from build123d import *

# Parameters (mm, degrees)
SKETCH_1_W          = 40
SKETCH_1_H          = 16.8
EXTRUDE_1_DEPTH     = 1
SKETCH_3_R          = 1.6
SKETCH_3_R_2        = 2.55
SKETCH_3_W          = 12.882492612
SKETCH_3_H          = 6.05
CUT_EXTRUDE_1_DEPTH = 2


with BuildPart() as part:
    # Эскиз1 → Бобышка-Вытянуть1 (new body)
    with BuildSketch(Plane(origin=(0, 0, 0), x_dir=(1, 0, 0), z_dir=(0, 1, 0))):
        Rectangle(SKETCH_1_W, SKETCH_1_H)
    extrude(amount=EXTRUDE_1_DEPTH)

    # Эскиз3 → Вырез-Вытянуть1 (cut, through all)
    with BuildSketch(Plane(origin=(0, 1, 0), x_dir=(1, 0, 0), z_dir=(0, 1, 0))):
        with Locations((-15, -3)):
            Circle(SKETCH_3_R)
        with Locations((15, -3)):
            Circle(SKETCH_3_R)
        with Locations((0, 2.35)):
            Circle(SKETCH_3_R_2)
        with Locations((13.558753694, 5.375)):
            Rectangle(SKETCH_3_W, SKETCH_3_H)
        with Locations((-13.558753694, 5.375)):
            Rectangle(SKETCH_3_W, SKETCH_3_H)
    extrude(amount=-CUT_EXTRUDE_1_DEPTH, mode=Mode.SUBTRACT)


solid = part.part
Read the model definition and answer for the solid it produces. Units are mm, in the model's axes. A direction names the side the tool comes from. Give positions to 0.01 mm unless a question says otherwise; leave off trailing zeros. Loops run counter-clockwise (first coordinate to the right, second up) from the corner with the lowest first, then second, coordinate; pieces in that order, holes last. Notation, with made-up numbers: (34.5, 58) -> (64.5, 58) arc R20 ccw to (64.5, 91) -> close; hole circle Ø1 at (-29.75, 27.5). An arc over 180 degrees is marked (long way). Use a Markdown table: item, result.
Q1. Section D-D, the plane z = -2.75 is taken. Determine the outline of the cut face in (x, y).
Solved:
| item | result |
|---|---|
| outline | (-7.12, 0) -> (-2.52, 0) -> (-2.52, 1) -> (-7.12, 1) -> close; (2.52, 0) -> (7.12, 0) -> (7.12, 1) -> (2.52, 1) -> close |
Q2. A tool of negligible diameter and unlimited length cuts with its end or side. For faces 1 (the face through (7.118, 0.5, -5.3)), 2 (the face through (-13.6, 0.5, -2.35)), 3 (the face through (0, 0, 2)), from which of +Z, -Z, +X, -X, +Y, -Y can it reach the whole face along a straight path? Write none if from no direction.
Solved:
| item | result |
|---|---|
| face 1 | -Z, +X, +Y, -Y |
| face 2 | -Z, -X, +Y, -Y |
| face 3 | +Z, -Z, +X, -X, -Y |
Q3. Section C-C, the plane y = 0.25 is taken. Determine the outline of the cut face in (x, z), then the cut area to 3 significant figures.
Solved:
| item | result |
|---|---|
| outline | (-20, -2.35) -> (-7.12, -2.35) -> (-7.12, -8.4) -> (7.12, -8.4) -> (7.12, -2.35) -> (20, -2.35) -> (20, 8.4) -> (-20, 8.4) -> close; hole circle Ø3.2 at (-15, 3); hole circle Ø5.1 at (0, -2.35); hole circle Ø3.2 at (15, 3) |
| area | 480 mm^2 |
Q4. Section A-A, the plane z = 3 is taken. Determine the outline of the cut face in (x, y).
Solved:
| item | result |
|---|---|
| outline | (-20, 0) -> (-16.6, 0) -> (-16.6, 1) -> (-20, 1) -> close; (-13.4, 0) -> (13.4, 0) -> (13.4, 1) -> (-13.4, 1) -> close; (16.6, 0) -> (20, 0) -> (20, 1) -> (16.6, 1) -> close |
Q5. Find the intervals of material crossed by line 1 along X through (y, z) = (0.7, 3); line 2 along Z through (x, y) = (15, 0.3); line 3 along Z through (x, y) = (0, 0.55), in increasing order.
Solved:
| item | result |
|---|---|
| line 1 | x = -20 to -16.6, -13.4 to 13.4, 16.6 to 20 |
| line 2 | z = -2.35 to 1.4, 4.6 to 8.4 |
| line 3 | z = -8.4 to -4.9, 0.2 to 8.4 |
Q6. Section B-B, the plane x = 15 is taken. Determine the outline of the cut face in (y, z).
Solved:
| item | result |
|---|---|
| outline | (0, -2.35) -> (1, -2.35) -> (1, 1.4) -> (0, 1.4) -> close; (0, 4.6) -> (1, 4.6) -> (1, 8.4) -> (0, 8.4) -> close |
